```python
from build123d import *

# Parameters (mm, degrees)
IZIM1_R                     = 25
Y_KSEKLIK_EKSTR_ZYON1_DEPTH = 18
IZIM2_R                     = 5
Y_KSEKLIK_EKSTR_ZYON2_DEPTH = 6
IZIM3_R                     = 10
Y_KSEKLIK_EKSTR_ZYON3_DEPTH = 7
IZIM4_R                     = 5
KES_EKSTR_ZYON1_DEPTH       = 7
IZIM9_R                     = 4
Y_KSEKLIK_EKSTR_ZYON5_DEPTH = 10
KES_EKSTR_ZYON2_DEPTH       = 16


with BuildPart() as part:
    # Çizim1 → Yükseklik-Ekstrüzyon1 (new body, symmetric)
    with BuildSketch(Plane(origin=(0, 0, 0), x_dir=(1, 0, 0), z_dir=(0, 1, 0))):
        Circle(IZIM1_R)
        with BuildLine():
            Line((-15.3, 4), (-11.313708499, 4))
            ThreePointArc((-11.313708499, 4), (12, 0), (-11.313708499, -4))
            Line((-11.313708499, -4), (-15.3, -4))
            Line((-15.3, -4), (-15.3, 4))
        make_face(mode=Mode.SUBTRACT)
    extrude(amount=Y_KSEKLIK_EKSTR_ZYON1_DEPTH, both=True)

    # Çizim2 → Yükseklik-Ekstrüzyon2 (add, symmetric)
    with BuildSketch(Plane(origin=(0, 0, 0), x_dir=(1, 0, 0), z_dir=(0, 1, 0))):
        with BuildLine():
            Line((-121.2, -8.919641248), (-3.333333333, -24.776781246))
            ThreePointArc((-3.333333333, -24.776781246), (-25, 0), (-3.333333333, 24.776781246))
            Line((-3.333333333, 24.776781246), (-121.2, 8.919641248))
            ThreePointArc((-121.2, 8.919641248), (-129, 0), (-121.2, -8.919641248))
        make_face()
        with Locations((-120, 0)):
            Circle(IZIM2_R, mode=Mode.SUBTRACT)
    extrude(amount=Y_KSEKLIK_EKSTR_ZYON2_DEPTH, both=True)

    # Çizim3 → Yükseklik-Ekstrüzyon3 (add)
    with BuildSketch(Plane(origin=(0, 6, 0), x_dir=(1, 0, 0), z_dir=(0, 1, 0))):
        with Locations((-48, 0)):
            Circle(IZIM3_R)
    extrude(amount=Y_KSEKLIK_EKSTR_ZYON3_DEPTH)

    # Çizim4 → Kes-Ekstrüzyon1 (cut)
    with BuildSketch(Plane(origin=(0, 13, 0), x_dir=(1, 0, 0), z_dir=(0, 1, 0))):
        with Locations((-48, 0)):
            Circle(IZIM4_R)
    extrude(amount=-KES_EKSTR_ZYON1_DEPTH, mode=Mode.SUBTRACT)

    # Çizim9 → Yükseklik-Ekstrüzyon5 (add, symmetric)
    with BuildSketch(Plane.XY):
        with BuildLine():
            Line((-76, 27), (-76, 6))
            Line((-76, 6), (-92, 6))
            Line((-92, 6), (-92, 27))
            ThreePointArc((-92, 27), (-84, 35), (-76, 27))
        make_face()
        with Locations((-84, 27)):
            Circle(IZIM9_R, mode=Mode.SUBTRACT)
    extrude(amount=Y_KSEKLIK_EKSTR_ZYON5_DEPTH, both=True)

    # Çizim10 → Kes-Ekstrüzyon2 (cut)
    with BuildSketch(Plane.ZY.offset(92)):
        Polygon((0, 6), (-2, 6), (-2, 27), (-2, 35), (0, 35), (0, 27), align=None)
    extrude(amount=-KES_EKSTR_ZYON2_DEPTH, mode=Mode.SUBTRACT)


solid = part.part
```
Could you check a few things on this model? Use its own coordinates, in mm. A direction names the side the tool comes from. Give positions to 0.01 mm unless a question says otherwise; leave off trailing zeros. Loops run counter-clockwise (first coordinate to the right, second up) from the corner with the lowest first, then second, coordinate; pieces in that order, holes last. Notation, with made-up numbers: (83, -32) -> (105, -32) arc R34 cw to (105, -1) -> close; hole circle Ø1 at (5, 54). An arc over 180 degrees is marked (long way). Put each result on its own line as item: value.
(1) Thinking about a two-plate mould opening in Y: for faces 1 (the face through (-92, 16, 5)), 2 (the face through (-48, 6, 0)), 3 (the face through (-86.95, 29.7, -6.06)), which applies, pulls with the +Y half, pulls with the -Y half, needs draft (parallel to the pull), parting line crosses it, or undercut?
Computed:
face 1: needs draft
face 2: pulls with the +Y half
face 3: undercut
(2) I'm going to push flat-ended pins straight in: pin 1 Ø5 at (y, z) = (-12, 8.5) entering from -X; pin 2 Ø3 at (x, z) = (-47, 0) entering from +Y; pin 3 Ø5 at (y, z) = (19.5, 2.5) entering from -X; pin 4 Ø6.5 at (x, y) = (-84, 27) entering from +Z. Where does each tip first touch, or does it pass through?
Computed:
pin 1: x = -24.27
pin 2: y = 6
pin 3: x = -92
pin 4: through
(3) Imagine slicing it at D-D on y = -12.5. Write out the boundary of the cut face in (x, z), plus the area to 3 significant figures.
Computed:
outline: circle Ø50 at (0, 0); hole (-15.3, -4) -> (-11.31, -4) arc R12 ccw (long way) to (-11.31, 4) -> (-15.3, 4) -> close
area: 1,480 mm^2
(4) Imagine slicing it at C-C on x = -84. Write out the boundary of the cut face in (y, z), plus the area to 3 significant figures.
Computed:
outline: (-6, -13.92) -> (6, -13.92) -> (6, -10) -> (23, -10) -> (23, -2) -> (6, -2) -> (6, 0) -> (23, 0) -> (23, 10) -> (6, 10) -> (6, 13.92) -> (-6, 13.92) -> close; (31, -10) -> (35, -10) -> (35, -2) -> (31, -2) -> close; (31, 0) -> (35, 0) -> (35, 10) -> (31, 10) -> close
area: 712 mm^2
(5) Please list where these lines run through material, in increasing order: probe 1 along X at (y, z) = (2.5, 0); probe 2 along Z at (x, y) = (0, 9); probe 3 along X at (y, z) = (2, -3). Write a range as [from, to].
Computed:
probe 1: [-129, -125], [-115, -15.3], [12, 25]
probe 2: [-25, -12], [12, 25]
probe 3: [-128.49, -124], [-116, -15.3], [11.62, 24.82]
(6) Imagine slicing it at B-B on z = 7.5. Write out the boundary of the cut face in (x, y).
Computed:
outline: (-124.97, -6) -> (-23.85, -6) -> (-23.85, -18) -> (-9.37, -18) -> (-9.37, 18) -> (-23.85, 18) -> (-23.85, 6) -> (-41.39, 6) -> (-41.39, 13) -> (-54.61, 13) -> (-54.61, 6) -> (-76, 6) -> (-76, 27) arc R8 ccw to (-92, 27) -> (-92, 6) -> (-124.97, 6) -> close; (9.37, -18) -> (23.85, -18) -> (23.85, 18) -> (9.37, 18) -> close; hole circle Ø8 at (-84, 27)
(7) Imagine slicing it at A-A on y = 7.5. Write out the boundary of the cut face in (x, z).
Computed:
outline: (-92, -10) -> (-76, -10) -> (-76, -2) -> (-92, -2) -> close; (-92, 0) -> (-76, 0) -> (-76, 10) -> (-92, 10) -> close; circle Ø20 at (-48, 0); circle Ø50 at (0, 0); hole circle Ø10 at (-48, 0); hole (-15.3, -4) -> (-11.31, -4) arc R12 ccw (long way) to (-11.31, 4) -> (-15.3, 4) -> close
(8) For faces 4 (the face through (-76, 17, 5)), 5 (the face through (-53, 10, 0)), 6 (the face through (-84, 17, 0)), 7 (the face through (-13, 0, -4)), 8 (the face through (23.846, 0.252, -7.509)), which set-ups out of +Z, -Z, +X, -X, +Y, -Y let a thin tool reach every point of the face, with its end or its side?
Computed:
face 4: +Z, -Z, +Y
face 5: +Y
face 6: -X, +Y
face 7: +Y, -Y
face 8: none
